Check sheet for the modelled part. Datum: model origin and axes. Units: mm. A direction names the side the tool comes from. Give positions to 0.01 mm unless a question says otherwise; leave off trailing zeros.
from build123d import *

# Parameters (mm, degrees)
SKETCH1_W                  = 84
SKETCH1_H                  = 55
EXTRUDE1_DEPTH             = 7
F_2_7_2_7_DIAMETER_HOLE1_D = 2.7
SKETCH6_OUTSIDE_W          = 106.13
SKETCH6_OUTSIDE_H          = 77.13
SKETCH6_OUTSIDE_R          = 2.5
EXTRUDE2_DEPTH             = 3
SKETCH7_W                  = 15
SKETCH7_H                  = 22
EXTRUDE3_DEPTH             = 1.1
SKETCH8_W                  = 26.471562954
SKETCH8_H                  = 62.575334395
SKETCH8_R                  = 2.5
EXTRUDE6_DEPTH             = 1
SKETCH9_W                  = 23
SKETCH9_H                  = 22
EXTRUDE7_DEPTH             = 0.6
M2_5X0_45_TAPPED_HOLE1_D   = 2.05
SKETCH14_W                 = 84
SKETCH14_H                 = 55
SKETCH14_R                 = 3
EXTRUDE12_DEPTH            = 5
SKETCH16_W                 = 105.280390668
SKETCH16_H                 = 3
EXTRUDE13_DEPTH            = 5


with BuildPart() as part:
    # Sketch1 → Extrude1 (new body)
    with BuildSketch(Plane.XY):
        Rectangle(SKETCH1_W, SKETCH1_H)
    extrude(amount=EXTRUDE1_DEPTH)

    # Ø2.7 (2.7) Diameter Hole1 (through all)
    with Locations(Plane.XY.offset(7)):
        with Locations((-38, 23.5), (38, 23.5), (38, -23.5), (-38, -23.5)):
            Hole(F_2_7_2_7_DIAMETER_HOLE1_D / 2)

    # Sketch6 outside → Extrude2 (cut)
    with BuildSketch(Plane.XY.offset(7)):
        Rectangle(SKETCH6_OUTSIDE_W, SKETCH6_OUTSIDE_H)
        with Locations((-38, 23.5)):
            Circle(SKETCH6_OUTSIDE_R, mode=Mode.SUBTRACT)
        with Locations((-38, -23.5)):
            Circle(SKETCH6_OUTSIDE_R, mode=Mode.SUBTRACT)
        with Locations((38, 23.5)):
            Circle(SKETCH6_OUTSIDE_R, mode=Mode.SUBTRACT)
        with Locations((38, -23.5)):
            Circle(SKETCH6_OUTSIDE_R, mode=Mode.SUBTRACT)
    extrude(amount=-EXTRUDE2_DEPTH, mode=Mode.SUBTRACT)

    # Sketch7 → Extrude3 (add)
    with BuildSketch(Plane.XY.offset(4)):
        with Locations((-14.5, 1.5)):
            Rectangle(SKETCH7_W, SKETCH7_H)
    extrude(amount=EXTRUDE3_DEPTH)

    # Sketch8 → Extrude6 (cut)
    with BuildSketch(Plane.XY.offset(4)):
        with Locations((-35.235781477, -1.105270853)):
            Rectangle(SKETCH8_W, SKETCH8_H)
        with Locations((-38, -23.5)):
            Circle(SKETCH8_R, mode=Mode.SUBTRACT)
        with Locations((-38, 23.5)):
            Circle(SKETCH8_R, mode=Mode.SUBTRACT)
    extrude(amount=-EXTRUDE6_DEPTH, mode=Mode.SUBTRACT)

    # Sketch9 → Extrude7 (add)
    with BuildSketch(Plane.XY.offset(4)):
        with Locations((4.5, 1.5)):
            Rectangle(SKETCH9_W, SKETCH9_H)
    extrude(amount=EXTRUDE7_DEPTH)

    # M2.5x0.45 Tapped Hole1 (through all)
    with Locations(Plane.XY.offset(7)):
        with Locations((-20.5, 20.5), (20.5, 20.5), (20.5, -20.5), (-20.5, -20.5)):
            Hole(M2_5X0_45_TAPPED_HOLE1_D / 2)

    # Sketch14 → Extrude12 (add)
    with BuildSketch(Plane(origin=(0, 0, 0), x_dir=(-1, 0, 0), z_dir=(0, 0, -1))):
        Rectangle(SKETCH14_W, SKETCH14_H)
        with Locations((-38, 23.5)):
            Circle(SKETCH14_R, mode=Mode.SUBTRACT)
        with Locations((-20.5, 20.5)):
            Circle(SKETCH14_R, mode=Mode.SUBTRACT)
        with Locations((20.5, 20.5)):
            Circle(SKETCH14_R, mode=Mode.SUBTRACT)
        with Locations((38, 23.5)):
            Circle(SKETCH14_R, mode=Mode.SUBTRACT)
        with Locations((-38, -23.5)):
            Circle(SKETCH14_R, mode=Mode.SUBTRACT)
        with Locations((-20.5, -20.5)):
            Circle(SKETCH14_R, mode=Mode.SUBTRACT)
        with Locations((20.5, -20.5)):
            Circle(SKETCH14_R, mode=Mode.SUBTRACT)
        with Locations((38, -23.5)):
            Circle(SKETCH14_R, mode=Mode.SUBTRACT)
    extrude(amount=EXTRUDE12_DEPTH)

    # Sketch16 → Extrude13 (cut)
    with BuildSketch(Plane(origin=(0, 0, -5), x_dir=(-1, 0, 0), z_dir=(0, 0, -1))):
        with Locations((-1.715862013, -22.499)):
            Rectangle(SKETCH16_W, SKETCH16_H)
        with Locations((-1.715862013, -17.499)):
            Rectangle(SKETCH16_W, SKETCH16_H)
        with Locations((-1.715862013, -12.499)):
            Rectangle(SKETCH16_W, SKETCH16_H)
        with Locations((-1.715862013, -7.499)):
            Rectangle(SKETCH16_W, SKETCH16_H)
        with Locations((-1.715862013, -2.499)):
            Rectangle(SKETCH16_W, SKETCH16_H)
        with Locations((-1.715862013, 2.501)):
            Rectangle(SKETCH16_W, SKETCH16_H)
        with Locations((-1.715862013, 7.501)):
            Rectangle(SKETCH16_W, SKETCH16_H)
        with Locations((-1.715862013, 12.501)):
            Rectangle(SKETCH16_W, SKETCH16_H)
        with Locations((-1.715862013, 17.501)):
            Rectangle(SKETCH16_W, SKETCH16_H)
        with Locations((-1.715862013, 22.501)):
            Rectangle(SKETCH16_W, SKETCH16_H)
    extrude(amount=-EXTRUDE13_DEPTH, mode=Mode.SUBTRACT)


solid = part.part
1) Sectioned sample at A-A on x = 38. Give the number of separate pieces and of enclosed holes in the cut face, then the cut area to 3 significant figures.
2) Scan lines: L1, parallel to Y at x = 38, z = 1.5; L2, parallel to X at y = 23.5, z = 2.5; L3, parallel to Y at x = -20.5, z = 1.75 (3 decimals). Record each from-to range of solid material in increasing order.
3) Gauge pin test, flat ends, axial feed: pin 1 (3 mm diameter, centred on y = -17, z = 5, fed in from -X); pin 2 (10 mm diameter, centred on x = 14.5, y = 18, fed in from +Z); pin 3 (6 mm diameter, centred on x = -30, y = -9.5, fed in from +Z). Record the tip position at first contact, or that the pin passes through.
4) Draft check along X on faces 1 (the flat face through (41, -20.999, -3)), 2 (the cylindrical face through (-20.367, -19.484, 1.972)). Enter one of: +X half, -X half, draft (parallel to the pull), parting line (faces both ways), or undercut.
5) Access from +Z, -Z, +X, -X, +Y, -Y to the whole of each face (thin tool, end or side, straight path). Record for faces 3 (the flat face through (1, -26, -5)), 4 (the cylindrical face through (39.34, -21.39, 5.52)), 5 (the cylindrical face through (-17.55, -19.95, -2.46)), 6 (the flat face through (0, 19.001, -3)).
Answers below:
1. separate pieces: 3
1. enclosed holes: 0
1. area: 307 mm2
2. L1: y = -27.5 to -24.85, -22.15 to 22.15, 24.85 to 27.5
2. L2: x = -42 to -39.35, -36.65 to 36.65, 39.35 to 42
2. L3: y = -27.5 to -21.525, -19.475 to 19.475, 21.525 to 27.5
3. pin 1: stops at x = -22
3. pin 2: stops at z = 4
3. pin 3: stops at z = 3
4. face 1: draft
4. face 2: undercut
5. face 3: -Z, +X, -X, +Y, -Y
5. face 4: +Z
5. face 5: -Z
5. face 6: -Z, +X, -X
